Answer from the drawing. Dimensions are ordinates in mm from the lowest x, y and z of the part. A direction names the side the tool comes from. Round coordinates to 2 decimals unless told otherwise and drop trailing zeros. Write each loop counter-clockwise with the first axis right and the second up, starting at its lowest first coordinate (ties: lowest second). Pieces come first, ordered by that corner, then holes. Notation, with made-up numbers: (45, 47.25) -> (54, 47.25) arc R15 cw to (54, 71.25) -> close; hole circle Ø10 at (31.5, 71.25). An arc over 180 degrees is marked (long way). Return JSON: item names as keys, results as strings. Group by question number.
(1) A cutting plane is placed at A-A on z = 36. Give the vertices of the cut face in (x, y).
(2) A cutting plane is placed at C-C on y = 9.5. Give the vertices of the cut face in (x, z).
(3) A cutting plane is placed at B-B on y = 41. Give the vertices of the cut face in (x, z), then the cut area to 3 significant figures.
(4) For the marked faces 1 and 2, determine the directions among +Z, -Z, +X, -X, +Y, -Y from which every point of the face is accessible in a straight line to the end or side of a thin tool.
(5) Given pin 1 (1.8 mm diameter, centred on x = 21, y = 41, fed in from +Z) (1 decimal); pin 2 (12 mm diameter, centred on x = 15.5, z = 27.5, fed in from +Y); pin 3 (1 mm diameter, centred on x = 9, y = 26, fed in from -Z), each flat-ended and moving along its own axis, determine where each tip first touches the part or whether it passes through.
(6) Straight lines are drawn through the part: line 1 (X direction, y = 0.8, z = 36); line 2 (Z direction, x = 2, y = 10); line 3 (Y direction, x = 36, z = 33.5). For each, find the intervals that lie inside material, in ascending order.
(7) A cutting plane is placed at D-D on y = 22. Give the vertices of the cut face in (x, z).
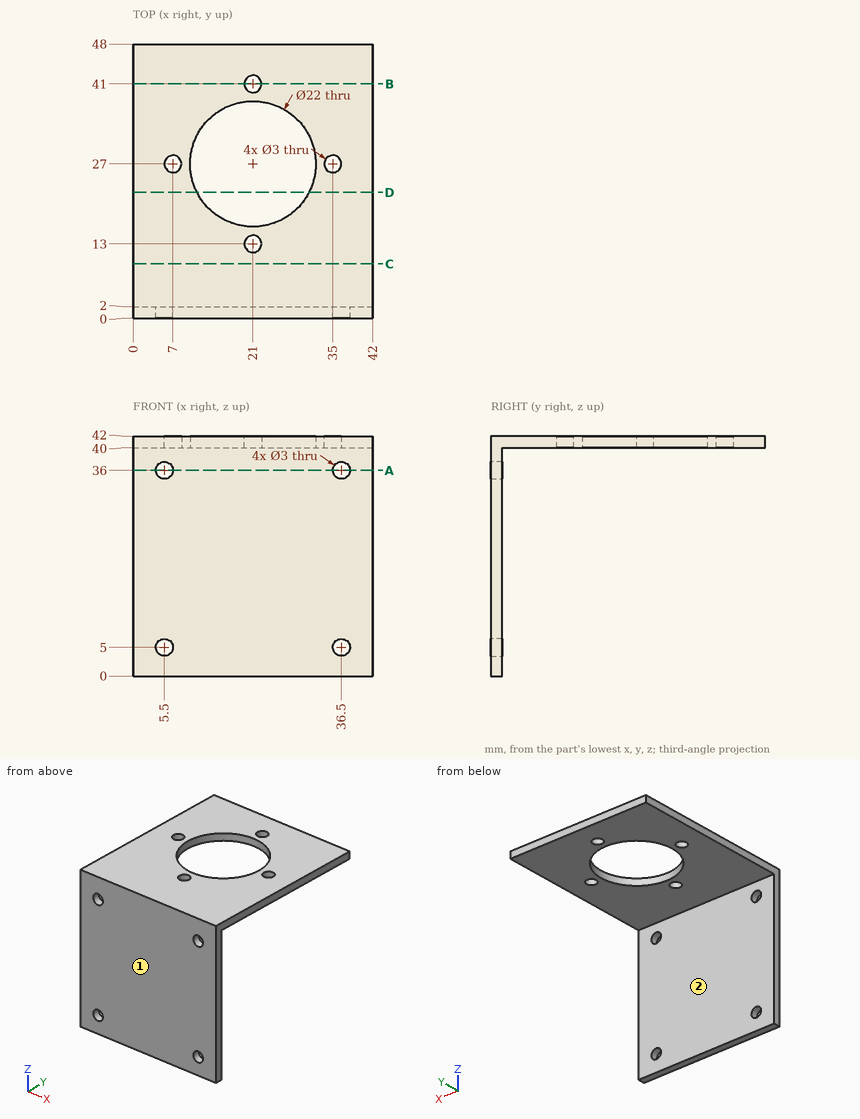
Checks:
{
 "1": {"outline": "(0, 0) -> (4, 0) -> (4, 2) -> (0, 2) -> close; (7, 0) -> (35, 0) -> (35, 2) -> (7, 2) -> close; (38, 0) -> (42, 0) -> (42, 2) -> (38, 2) -> close"},
 "2": {"outline": "(0, 40) -> (42, 40) -> (42, 42) -> (0, 42) -> close"},
 "3": {"outline": "(0, 40) -> (19.5, 40) -> (19.5, 42) -> (0, 42) -> close; (22.5, 40) -> (42, 40) -> (42, 42) -> (22.5, 42) -> close", "area": "78.0 mm^2"},
 "4": {"face 1": "+Z, -Z, +X, -X, -Y", "face 2": "-Z, +X, -X, +Y"},
 "5": {"pin 1": "passes through", "pin 2": "stops at y = 2", "pin 3": "stops at z = 40"},
 "6": {"line 1": "x = 0 to 4, 7 to 35, 38 to 42", "line 2": "z = 40 to 42", "line 3": "y = 0 to 2"},
 "7": {"outline": "(0, 40) -> (11.2, 40) -> (11.2, 42) -> (0, 42) -> close; (30.8, 40) -> (42, 40) -> (42, 42) -> (30.8, 42) -> close"}
}
